from build123d import *

# Parameters (mm, degrees)
SKETCH1_R                 = 2.54
SKETCH1_R_2               = 1.905
BOSS_EXTRUDE1_DEPTH       = 10.922
BOSS_EXTRUDE1_2_DEPTH     = 10.922
BOSS_EXTRUDE1_3_DEPTH     = 10.922
BOSS_EXTRUDE1_4_DEPTH     = 10.922
BOSS_EXTRUDE3_START       = -10.922
BOSS_EXTRUDE3_OUTLINE_R   = 1.905
BOSS_EXTRUDE3_DEPTH       = 10.922
BOSS_EXTRUDE3_2_OUTLINE_R = 1.905
BOSS_EXTRUDE3_2_DEPTH     = 10.922
BOSS_EXTRUDE3_3_OUTLINE_R = 1.905
BOSS_EXTRUDE3_3_DEPTH     = 10.922
BOSS_EXTRUDE3_4_OUTLINE_R = 1.905
BOSS_EXTRUDE3_4_DEPTH     = 10.922
BOSS_EXTRUDE4_START       = 4.318
SKETCH3_R                 = 1.905
BOSS_EXTRUDE4_DEPTH       = 4.318
FILLET1_R                 = 6.35
CUT_EXTRUDE1_REACH        = 176.845
SKETCH5_R                 = 2.159


with BuildPart() as part:
    # Sketch1 → Boss-Extrude1 (new body)
    with BuildSketch(Plane.XY):
        with Locations((83.701311305, -41.752062977)):
            Circle(SKETCH1_R)
        with Locations((83.701311305, -41.752062977)):
            Circle(SKETCH1_R_2, mode=Mode.SUBTRACT)
    extrude(amount=-BOSS_EXTRUDE1_DEPTH)

    # Boss-Extrude3: read off the stored shape, not the designer's step
    # Boss-Extrude3 outline → Boss-Extrude3 (add)
    with BuildSketch(Plane.XY.offset(BOSS_EXTRUDE3_START)):
        with BuildLine():
            Line((89.670311305, -35.783062977), (76.540111305, -35.783062977))
            ThreePointArc((76.540111305, -35.783062977), (81.82257698, -43.469198406), (89.670311305, -48.508462977))
            Line((89.670311305, -48.508462977), (89.670311305, -35.783062977))
        make_face()
        with Locations((83.701311305, -41.752062977)):
            Circle(BOSS_EXTRUDE3_OUTLINE_R, mode=Mode.SUBTRACT)
    extrude(amount=BOSS_EXTRUDE3_DEPTH)



with BuildPart() as body_2:
    # Sketch1 → Boss-Extrude1 2 (new body)
    with BuildSketch(Plane.XY):
        with Locations((-14.088688695, -41.752062977)):
            Circle(SKETCH1_R)
        with Locations((-14.088688695, -41.752062977)):
            Circle(SKETCH1_R_2, mode=Mode.SUBTRACT)
    extrude(amount=-BOSS_EXTRUDE1_2_DEPTH)

    # Boss-Extrude3 4 outline → Boss-Extrude3 4 (add)
    with BuildSketch(Plane.XY.offset(BOSS_EXTRUDE3_START)):
        with BuildLine():
            Line((-20.057688695, -35.783062977), (-20.057688695, -46.006562977))
            ThreePointArc((-20.057688695, -46.006562977), (-12.297393991, -43.552911895), (-9.874167768, -35.783062977))
            Line((-9.874167768, -35.783062977), (-20.057688695, -35.783062977))
        make_face()
        with Locations((-14.088688695, -41.752062977)):
            Circle(BOSS_EXTRUDE3_4_OUTLINE_R, mode=Mode.SUBTRACT)
    extrude(amount=BOSS_EXTRUDE3_4_DEPTH)


with BuildPart() as body_3:
    # Sketch1 → Boss-Extrude1 3 (new body)
    with BuildSketch(Plane.XY):
        with Locations((-14.088688695, -135.732062977)):
            Circle(SKETCH1_R)
        with Locations((-14.088688695, -135.732062977)):
            Circle(SKETCH1_R_2, mode=Mode.SUBTRACT)
    extrude(amount=-BOSS_EXTRUDE1_3_DEPTH)

    # Boss-Extrude3 3 outline → Boss-Extrude3 3 (add)
    with BuildSketch(Plane.XY.offset(BOSS_EXTRUDE3_START)):
        with BuildLine():
            Line((-20.057688695, -141.701062977), (-6.875088695, -141.701062977))
            ThreePointArc((-6.875088695, -141.701062977), (-12.276682873, -133.951830584), (-20.057688695, -128.59610741))
            Line((-20.057688695, -128.59610741), (-20.057688695, -141.701062977))
        make_face()
        with Locations((-14.088688695, -135.732062977)):
            Circle(BOSS_EXTRUDE3_3_OUTLINE_R, mode=Mode.SUBTRACT)
    extrude(amount=BOSS_EXTRUDE3_3_DEPTH)


with BuildPart() as body_4:
    # Sketch1 → Boss-Extrude1 4 (new body)
    with BuildSketch(Plane.XY):
        with Locations((83.701311305, -135.732062977)):
            Circle(SKETCH1_R)
        with Locations((83.701311305, -135.732062977)):
            Circle(SKETCH1_R_2, mode=Mode.SUBTRACT)
    extrude(amount=-BOSS_EXTRUDE1_4_DEPTH)

    # Boss-Extrude3 2 outline → Boss-Extrude3 2 (add)
    with BuildSketch(Plane.XY.offset(BOSS_EXTRUDE3_START)):
        with BuildLine():
            Line((89.670311305, -141.701062977), (89.670311305, -132.150662977))
            ThreePointArc((89.670311305, -132.150662977), (80.369588205, -134.573287653), (73.922311305, -141.701062977))
            Line((73.922311305, -141.701062977), (89.670311305, -141.701062977))
        make_face()
        with Locations((83.701311305, -135.732062977)):
            Circle(BOSS_EXTRUDE3_2_OUTLINE_R, mode=Mode.SUBTRACT)
    extrude(amount=BOSS_EXTRUDE3_2_DEPTH)


with BuildPart() as part_1:
    add(part.part)

    add(body_2.part)  # Boss-Extrude4 merges body 2

    add(body_3.part)  # Boss-Extrude4 merges body 3

    add(body_4.part)  # Boss-Extrude4 merges body 4
    # Sketch3 → Boss-Extrude4 (add)
    with BuildSketch(Plane.XY.offset(BOSS_EXTRUDE4_START)):
        with BuildLine():
            Line((-24.756688695, -101.757891635), (-24.756688695, -146.400062977))
            Line((-24.756688695, -146.400062977), (94.369311305, -146.400062977))
            Line((94.369311305, -146.400062977), (94.369311305, -101.676974724))
            ThreePointArc((94.369311305, -101.676974724), (90.432311305, -96.933562977), (94.369311305, -92.19015123))
            Line((94.369311305, -92.19015123), (94.369311305, -62.814974724))
            ThreePointArc((94.369311305, -62.814974724), (90.432311305, -58.071562977), (94.369311305, -53.32815123))
            Line((94.369311305, -53.32815123), (94.369311305, -31.084062977))
            Line((94.369311305, -31.084062977), (-24.756688695, -31.084062977))
            Line((-24.756688695, -31.084062977), (-24.756688695, -53.882487661))
            ThreePointArc((-24.756688695, -53.882487661), (-20.438688695, -58.071562977), (-24.756688695, -62.260638293))
            Line((-24.756688695, -62.260638293), (-24.756688695, -92.109234319))
            ThreePointArc((-24.756688695, -92.109234319), (-19.803688695, -96.933562977), (-24.756688695, -101.757891635))
        make_face()
        with Locations((83.701311305, -41.752062977)):
            Circle(SKETCH3_R, mode=Mode.SUBTRACT)
        with Locations((-14.088688695, -135.732062977)):
            Circle(SKETCH3_R, mode=Mode.SUBTRACT)
        with Locations((83.701311305, -135.732062977)):
            Circle(SKETCH3_R, mode=Mode.SUBTRACT)
        with Locations((-14.088688695, -41.752062977)):
            Circle(SKETCH3_R, mode=Mode.SUBTRACT)
    extrude(amount=-BOSS_EXTRUDE4_DEPTH)

    # Fillet1
    fillet1_edges = [part_1.edges().sort_by_distance(p)[0] for p in [
        (-24.756688695, -146.400062977, 2.159),
        (94.369311305, -146.400062977, 2.159),
        (94.369311305, -31.084062977, 2.159),
        (-24.756688695, -31.084062977, 2.159),
    ]]
    fillet(fillet1_edges, radius=FILLET1_R)

    # Sketch5 → Cut-Extrude1 (cut, up to next)
    with BuildSketch(Plane.XY.offset(4.318), mode=Mode.PRIVATE) as cut_extrude1_sk1:
        with BuildLine():
            Line((5.850311305, -98.140062977), (34.806311305, -98.140062977))
            Line((34.806311305, -98.140062977), (34.806311305, -69.184062977))
            Line((34.806311305, -69.184062977), (20.021852978, -69.184062977))
            ThreePointArc((20.021852978, -69.184062977), (11.816855635, -75.150607307), (5.850311305, -83.355604651))
            Line((5.850311305, -83.355604651), (5.850311305, -98.140062977))
        make_face()
    cut_extrude1_tool1 = extrude(cut_extrude1_sk1.sketch, amount=-CUT_EXTRUDE1_REACH, mode=Mode.PRIVATE) & part_1.part
    # Sketch5 → Cut-Extrude1 (cut, up to next)
    with BuildSketch(Plane.XY.offset(4.318), mode=Mode.PRIVATE) as cut_extrude1_sk2:
        with BuildLine():
            Line((34.806311305, -69.184062977), (34.806311305, -98.140062977))
            Line((34.806311305, -98.140062977), (63.762311305, -98.140062977))
            Line((63.762311305, -98.140062977), (63.762311305, -83.355604651))
            ThreePointArc((63.762311305, -83.355604651), (57.795766975, -75.150607307), (49.590769631, -69.184062977))
            Line((49.590769631, -69.184062977), (34.806311305, -69.184062977))
        make_face()
    cut_extrude1_tool2 = extrude(cut_extrude1_sk2.sketch, amount=-CUT_EXTRUDE1_REACH, mode=Mode.PRIVATE) & part_1.part
    # Sketch5 → Cut-Extrude1 (cut, up to next)
    with BuildSketch(Plane.XY.offset(4.318), mode=Mode.PRIVATE) as cut_extrude1_sk3:
        with Locations((9.787309036, -73.121060708)):
            Circle(SKETCH5_R)
    cut_extrude1_tool3 = extrude(cut_extrude1_sk3.sketch, amount=-CUT_EXTRUDE1_REACH, mode=Mode.PRIVATE) & part_1.part
    # Sketch5 → Cut-Extrude1 (cut, up to next)
    with BuildSketch(Plane.XY.offset(4.318), mode=Mode.PRIVATE) as cut_extrude1_sk4:
        with Locations((59.825309036, -73.121065246)):
            Circle(SKETCH5_R)
    cut_extrude1_tool4 = extrude(cut_extrude1_sk4.sketch, amount=-CUT_EXTRUDE1_REACH, mode=Mode.PRIVATE) & part_1.part
    # Sketch5 → Cut-Extrude1 (cut, up to next)
    with BuildSketch(Plane.XY.offset(4.318), mode=Mode.PRIVATE) as cut_extrude1_sk5:
        with Locations((59.825313573, -123.159065246)):
            Circle(SKETCH5_R)
    cut_extrude1_tool5 = extrude(cut_extrude1_sk5.sketch, amount=-CUT_EXTRUDE1_REACH, mode=Mode.PRIVATE) & part_1.part
    # Sketch5 → Cut-Extrude1 (cut, up to next)
    with BuildSketch(Plane.XY.offset(4.318), mode=Mode.PRIVATE) as cut_extrude1_sk6:
        with BuildLine():
            Line((34.806311305, -98.140062977), (34.806311305, -127.096062977))
            Line((34.806311305, -127.096062977), (49.590769631, -127.096062977))
            ThreePointArc((49.590769631, -127.096062977), (57.795766975, -121.129518647), (63.762311305, -112.924521303))
            Line((63.762311305, -112.924521303), (63.762311305, -98.140062977))
            Line((63.762311305, -98.140062977), (34.806311305, -98.140062977))
        make_face()
    cut_extrude1_tool6 = extrude(cut_extrude1_sk6.sketch, amount=-CUT_EXTRUDE1_REACH, mode=Mode.PRIVATE) & part_1.part
    # Sketch5 → Cut-Extrude1 (cut, up to next)
    with BuildSketch(Plane.XY.offset(4.318), mode=Mode.PRIVATE) as cut_extrude1_sk7:
        with BuildLine():
            Line((20.021852978, -127.096062977), (34.806311305, -127.096062977))
            Line((34.806311305, -127.096062977), (34.806311305, -98.140062977))
            Line((34.806311305, -98.140062977), (5.850311305, -98.140062977))
            Line((5.850311305, -98.140062977), (5.850311305, -112.924521303))
            ThreePointArc((5.850311305, -112.924521303), (11.816855635, -121.129518647), (20.021852978, -127.096062977))
        make_face()
    cut_extrude1_tool7 = extrude(cut_extrude1_sk7.sketch, amount=-CUT_EXTRUDE1_REACH, mode=Mode.PRIVATE) & part_1.part
    # Sketch5 → Cut-Extrude1 (cut, up to next)
    with BuildSketch(Plane.XY.offset(4.318), mode=Mode.PRIVATE) as cut_extrude1_sk8:
        with Locations((9.787313573, -123.159060708)):
            Circle(SKETCH5_R)
    cut_extrude1_tool8 = extrude(cut_extrude1_sk8.sketch, amount=-CUT_EXTRUDE1_REACH, mode=Mode.PRIVATE) & part_1.part
    add(cut_extrude1_tool1.solids().sort_by_distance((21.39883, -84.732582, 4.318))[0], mode=Mode.SUBTRACT)
    add(cut_extrude1_tool2.solids().sort_by_distance((48.213793, -84.732582, 4.318))[0], mode=Mode.SUBTRACT)
    add(cut_extrude1_tool3.solids().sort_by_distance((9.787309, -73.121061, 4.318))[0], mode=Mode.SUBTRACT)
    add(cut_extrude1_tool4.solids().sort_by_distance((59.825309, -73.121065, 4.318))[0], mode=Mode.SUBTRACT)
    add(cut_extrude1_tool5.solids().sort_by_distance((59.825314, -123.159065, 4.318))[0], mode=Mode.SUBTRACT)
    add(cut_extrude1_tool6.solids().sort_by_distance((48.213793, -111.547544, 4.318))[0], mode=Mode.SUBTRACT)
    add(cut_extrude1_tool7.solids().sort_by_distance((21.39883, -111.547544, 4.318))[0], mode=Mode.SUBTRACT)
    add(cut_extrude1_tool8.solids().sort_by_distance((9.787314, -123.159061, 4.318))[0], mode=Mode.SUBTRACT)


solid = part_1.part
Verification items for the finished model (mm, model axes). A direction names the side the tool comes from. Give positions to 0.01 mm unless a question says otherwise; leave off trailing zeros. Loops run counter-clockwise (first coordinate to the right, second up) from the corner with the lowest first, then second, coordinate; pieces in that order, holes last.
1) Sectioned sample at B-B, the plane z = -8.25. Enter the section's corners in (x, y) (3 decimals).
2) Thickness scan on line 1 along Y through (x, z) = (44.5, 0.5); line 2 along X through (y, z) = (-123.5, 3); line 3 along X through (y, z) = (-122, 3). Record the ranges inside material, lowest first.
3) Set-up check for faces 5 (the cylindrical face through (11.72, -121.03, 2.19)), 6 (the cylindrical face through (81.73, -43.38, -5.54)), 7 (the flat face through (-14, -141.701, -6)), 8 (the flat face through (83, -138, -10.922)): record each of +Z, -Z, +X, -X, +Y, -Y from which the full face is reachable in a straight line by a thin tool's end or side.
4) Sectioned sample at A-A, the plane x = 26. Enter the section's corners in (y, z), then the cut area to 3 significant figures.
5) Depth check by flat-ended pin: pin 1 Ø3.5 at (x, z) = (-14, -8) entering from -Y; pin 2 Ø5 at (x, y) = (76, -103) entering from -Z; pin 3 Ø3 at (y, z) = (-43, -7.5) entering from -X; pin 4 Ø3.5 at (x, y) = (9.79, -73.12) entering from -Z. Enter the tip coordinate at first touch or a pass-through.
6) Draft check along X on faces 1 (the flat face through (89.67, -42, -6)), 2 (the cylindrical face through (59.54, -121.02, 2.19)), 3 (the flat face through (35, -69.184, 2)), 4 (the flat face through (-20.058, -41, -6)). Enter one of: pulls with the +X half, pulls with the -X half, needs draft (parallel to the pull), parting line crosses it, or undercut.
7) Sectioned sample at C-C, the plane x = 67.5. Enter the section's corners in (y, z), then the cut area to 3 significant figures.
Answers:
1. outline: (-20.058, -141.701) - (-6.875, -141.701) arc R26.438 ccw to (-20.058, -128.596) - close; (-20.058, -46.007) arc R8.794 ccw to (-9.874, -35.783) - (-20.058, -35.783) - close; (73.922, -141.701) - (89.67, -141.701) - (89.67, -132.151) arc R16.787 ccw to start; (76.54, -35.783) arc R23.598 ccw to (89.67, -48.508) - (89.67, -35.783) - close; hole circle Ø3.81 at (-14.089, -135.732); hole circle Ø3.81 at (-14.089, -41.752); hole circle Ø3.81 at (83.701, -135.732); hole circle Ø3.81 at (83.701, -41.752)
2. line 1: y = -146.4 to -127.1, -69.18 to -31.08
2. line 2: x = -24.76 to 7.66, 11.92 to 14.46, 55.15 to 57.69, 61.96 to 94.37
2. line 3: x = -24.76 to 7.97, 11.61 to 12.72, 56.89 to 58, 61.65 to 94.37
3. face 5: +Z, -Z
3. face 6: -Z
3. face 7: -Z, +X, -X, -Y
3. face 8: -Z, +X, -X, +Y, -Y
4. outline: (-146.4, 0) - (-127.1, 0) - (-127.1, 4.32) - (-146.4, 4.32) - close; (-69.18, 0) - (-31.08, 0) - (-31.08, 4.32) - (-69.18, 4.32) - close
4. area: 248 mm2
5. pin 1: stops at y = -141.7
5. pin 2: stops at z = 0
5. pin 3: stops at x = -20.06
5. pin 4: passes through
6. face 1: pulls with the +X half
6. face 2: undercut
6. face 3: undercut
6. face 4: pulls with the -X half
7. outline: (-146.4, 0) - (-31.08, 0) - (-31.08, 4.32) - (-146.4, 4.32) - close
7. area: 498 mm2
